Verification items for the finished model (mm, model axes). A direction names the side the tool comes from. Coordinates: 2 decimals unless noted, no trailing zeros. Write each loop counter-clockwise with the first axis right and the second up, starting at its lowest first coordinate (ties: lowest second). Pieces come first, ordered by that corner, then holes. Notation, with made-up numbers: M 4.5,54.25 L 14.5,54.25 A28 cw 14.5,73.25 Z; hole C 85.25,88 d1. An arc over 180 degrees is marked long. One line per item, written item: value.
```python
from build123d import *
from build123d.topology import SkipClean

# Parameters (mm, degrees)
BASPROSKE_W         = 26
BASPROSKE_H         = 4.375
TOOTHCUT_DEPTH      = 60.063525123
TEETHCUTS_COUNT     = 55
TEETHCUTS_ANGLE     = 353.454545455
SKETCH2_R           = 37.5
BOSS_EXTRUDE2_DEPTH = 4.5
SKETCH3_R           = 2.25
SKETCH3_R_2         = 1.8
CUT_EXTRUDE1_DEPTH  = 4.5
SKETCH4_R           = 3.25
CUT_EXTRUDE2_DEPTH  = 3
BOSS_EXTRUDE3_START = 4
SKETCH5_R           = 37.5
SKETCH5_R_2         = 28.5
BOSS_EXTRUDE3_DEPTH = 4
BOSS_EXTRUDE4_START = 7
SKETCH6_R           = 37.5
SKETCH6_R_2         = 32.75
BOSS_EXTRUDE4_DEPTH = 7
SKETCH7_R           = 1.65
BOSS_EXTRUDE5_DEPTH = 10
FILLET1_R           = 3
BOSS_EXTRUDE6_START = -10
SKETCH8_R           = 1.65
BOSS_EXTRUDE6_DEPTH = 10
FILLET2_R           = 3
SKETCH9_R           = 37.6
SKETCH9_R_2         = 37.5
BOSS_EXTRUDE7_DEPTH = 10
FILLET3_R           = 3
SKETCH10_R          = 45.899134002
SKETCH10_R_2        = 2.25
CUT_EXTRUDE3_DEPTH  = 31.5
SKETCH12_R          = 1.65
SKETCH12_R_2        = 28.5
BOSS_EXTRUDE8_DEPTH = 1.15


with BuildPart() as part:
    # BasProSke → Base-Revolve (revolve)
    with BuildSketch(Plane(origin=(0, 0, 0), x_dir=(1, 0, 0), z_dir=(0, 1, 0)), mode=Mode.PRIVATE) as base_revolve_sk:
        with Locations((13, 35.3125)):
            Rectangle(BASPROSKE_W, BASPROSKE_H)
    revolve(base_revolve_sk.sketch.rotate(Axis((-10, 0, 0), (1, 0, 0)), 180), axis=Axis((-10, 0, 0), (1, 0, 0)))

    # TooCutSke → ToothCut (cut, through all)
    with BuildSketch(Plane(origin=(0, 0, 0), x_dir=(0, 0, -1), z_dir=(1, 0, 0))):
        with BuildLine():
            ThreePointArc((1.451447951, 33.067761022), (1.040603726, 34.522224287), (0.503573985, 35.934971761))
            ThreePointArc((0.503573985, 35.934971761), (0, 35.9385), (-0.503573985, 35.934971761))
            ThreePointArc((-0.503573985, 35.934971761), (-1.040603726, 34.522224287), (-1.451447951, 33.067761022))
            ThreePointArc((-1.451447951, 33.067761022), (0, 33.0996), (1.451447951, 33.067761022))
        make_face()
    toothcut = extrude(amount=TOOTHCUT_DEPTH, mode=Mode.SUBTRACT)

    # TeethCuts: ToothCut ×55 about axis
    teethcuts_axis = Axis((-10, 0, 0), (1, 0, 0))
    for i in range(1, TEETHCUTS_COUNT):
        add(toothcut.rotate(teethcuts_axis, i * TEETHCUTS_ANGLE / (TEETHCUTS_COUNT - 1)), mode=Mode.SUBTRACT)

    # Sketch2 → Boss-Extrude2 (add)
    with BuildSketch(Plane.ZY):
        Circle(SKETCH2_R)
    extrude(amount=BOSS_EXTRUDE2_DEPTH)

    # Sketch3 → Cut-Extrude1 (cut)
    with BuildSketch(Plane.ZY.offset(4.5)):
        Circle(SKETCH3_R)
        with Locations((0, 8.5)):
            Circle(SKETCH3_R_2)
        with Locations(Location((0, -8.5, 0), (0, 0, 180))):
            Circle(SKETCH3_R_2)
    extrude(amount=-CUT_EXTRUDE1_DEPTH, mode=Mode.SUBTRACT)

    # Sketch4 → Cut-Extrude2 (cut)
    with BuildSketch(Plane(origin=(0, 0, 0), x_dir=(0, 0, -1), z_dir=(1, 0, 0))):
        with Locations((0, -8.5)):
            Circle(SKETCH4_R)
        with Locations((0, 8.5)):
            Circle(SKETCH4_R)
    extrude(amount=-CUT_EXTRUDE2_DEPTH, mode=Mode.SUBTRACT)

    # Sketch5 → Boss-Extrude3 (add)
    with BuildSketch(Plane(origin=(26, 0, 0), x_dir=(0, 0, -1), z_dir=(1, 0, 0)).offset(BOSS_EXTRUDE3_START)):
        with Locations(Location((0, 0, 0), (0, 0, 180))):
            Circle(SKETCH5_R)
        Circle(SKETCH5_R_2, mode=Mode.SUBTRACT)
    extrude(amount=-BOSS_EXTRUDE3_DEPTH)

    # Sketch6 → Boss-Extrude4 (add)
    with BuildSketch(Plane(origin=(30, 0, 0), x_dir=(0, 0, -1), z_dir=(1, 0, 0)).offset(BOSS_EXTRUDE4_START)):
        with Locations(Location((0, 0, 0), (0, 0, 180))):
            Circle(SKETCH6_R)
        Circle(SKETCH6_R_2, mode=Mode.SUBTRACT)
    extrude(amount=-BOSS_EXTRUDE4_DEPTH)

    # Sketch7 → Boss-Extrude5 (add)
    # profile 1 of 3: a face of its own
    with BuildSketch(Plane(origin=(37, 0, 0), x_dir=(0, 0, -1), z_dir=(1, 0, 0))):
        with BuildLine():
            ThreePointArc((-30.713496008, 21.515835168), (-39.750566034, 22.95), (-33.990007843, 15.840750198))
            ThreePointArc((-33.990007843, 15.840750198), (-32.475952642, 18.75), (-30.713496008, 21.515835168))
        make_face()
        with Locations((-35.507041555, 20.5)):
            Circle(SKETCH7_R, mode=Mode.SUBTRACT)
    # profile 2 of 3: a face of its own
    with BuildSketch(Plane(origin=(37, 0, 0), x_dir=(0, 0, -1), z_dir=(1, 0, 0))):
        with BuildLine():
            ThreePointArc((-3.276511835, -37.356585366), (0, -45.9), (3.276511835, -37.356585366))
            ThreePointArc((3.276511835, -37.356585366), (0, -37.5), (-3.276511835, -37.356585366))
        make_face()
        with Locations((0, -41)):
            Circle(SKETCH7_R, mode=Mode.SUBTRACT)
    # profile 3 of 3: a face of its own
    with BuildSketch(Plane(origin=(37, 0, 0), x_dir=(0, 0, -1), z_dir=(1, 0, 0))):
        with BuildLine():
            ThreePointArc((30.713496008, 21.515835168), (32.475952642, 18.75), (33.990007843, 15.840750198))
            ThreePointArc((33.990007843, 15.840750198), (39.750566034, 22.95), (30.713496008, 21.515835168))
        make_face()
        with Locations((35.507041555, 20.5)):
            Circle(SKETCH7_R, mode=Mode.SUBTRACT)
    extrude(amount=-BOSS_EXTRUDE5_DEPTH)

    # Fillet1
    fillet1_edges = [part.edges().sort_by_distance(p)[0] for p in [
        (32, 15.840750198, 33.990007843),
        (32, 21.515835168, 30.713496008),
        (32, -37.356585366, -3.276511835),
        (32, -37.356585366, 3.276511835),
        (32, 21.515835168, -30.713496008),
        (32, 15.840750198, -33.990007843),
    ]]
    fillet(fillet1_edges, radius=FILLET1_R)

    # Sketch8 → Boss-Extrude6 (add)
    # profile 1 of 3: a face of its own
    with BuildSketch(Plane.ZY.offset(4.5).offset(BOSS_EXTRUDE6_START)):
        with BuildLine():
            ThreePointArc((3.277032239, 37.357537298), (-0.001858552, 45.899133961), (-3.279499265, 37.357057531))
            ThreePointArc((-3.279499265, 37.357057531), (-0.001244018, 37.500865925), (3.277032239, 37.357537298))
        make_face()
        with Locations((0, 41)):
            Circle(SKETCH8_R, mode=Mode.SUBTRACT)
    # profile 2 of 3: a face of its own
    with BuildSketch(Plane.ZY.offset(4.5).offset(BOSS_EXTRUDE6_START)):
        with BuildLine():
            ThreePointArc((30.71426819, -21.517740103), (39.750655671, -22.948112687), (33.993202634, -15.837979147))
            ThreePointArc((33.993202634, -15.837979147), (32.478138639, -18.749677793), (30.71426819, -21.517740103))
        make_face()
        with Locations((35.507041555, -20.5)):
            Circle(SKETCH8_R, mode=Mode.SUBTRACT)
    # profile 3 of 3: a face of its own
    with BuildSketch(Plane.ZY.offset(4.5).offset(BOSS_EXTRUDE6_START)):
        with BuildLine():
            ThreePointArc((-30.712203543, -21.517680022), (-32.47526663, -18.751188157), (-33.989800256, -15.841195617))
            ThreePointArc((-33.989800256, -15.841195617), (-39.748976395, -22.951021278), (-30.712203543, -21.517680022))
        make_face()
        with Locations((-35.507041555, -20.5)):
            Circle(SKETCH8_R, mode=Mode.SUBTRACT)
    extrude(amount=BOSS_EXTRUDE6_DEPTH)


with BuildPart() as boss_extrude6_piece_1:
    # of the separate pieces the step leaves, piece 1, a body of its own (boss_extrude6_pieces)
    add(part.part.solids().sort_by_distance((37, -36.798102981, 7.221469172))[0])

    # Fillet2
    fillet2_edges = [boss_extrude6_piece_1.edges().sort_by_distance(p)[0] for p in [
        (0.5, -21.517680022, -30.712203543),
        (0.5, -15.841195617, -33.989800256),
    ]]
    fillet(fillet2_edges, radius=FILLET2_R)



with BuildPart() as boss_extrude6_piece_2:
    # of the separate pieces the step leaves, piece 2, a body of its own (boss_extrude6_pieces)
    add(part.part.solids().sort_by_distance((5.5, 37.357057531, -3.279499265))[0])


with BuildPart() as boss_extrude6_piece_3:
    # of the separate pieces the step leaves, piece 3, a body of its own (boss_extrude6_pieces)
    add(part.part.solids().sort_by_distance((5.5, -15.837979147, 33.993202634))[0])


with BuildPart() as boss_extrude6_piece_1_1:
    add(boss_extrude6_piece_1.part)

    add(boss_extrude6_piece_2.part)  # Boss-Extrude7 merges Boss-Extrude6 piece 2

    add(boss_extrude6_piece_3.part)  # Boss-Extrude7 merges Boss-Extrude6 piece 3
    # Sketch9 → Boss-Extrude7 (add)
    with BuildSketch(Plane.ZY.offset(4.5)):
        Circle(SKETCH9_R)
        Circle(SKETCH9_R_2, mode=Mode.SUBTRACT)
    extrude(amount=-BOSS_EXTRUDE7_DEPTH)

    # Fillet3
    fillet3_edges = [boss_extrude6_piece_1_1.edges().sort_by_distance(p)[0] for p in [
        (0.5, 37.448219223, 3.375037342),
        (0.5, 37.447972163, -3.377777505),
        (0.5, -21.646977688, 30.743590502),
        (0.5, -15.798744954, 34.119783966),
    ]]
    fillet(fillet3_edges, radius=FILLET3_R)

    # Sketch10 → Cut-Extrude3 (cut)
    with BuildSketch(Plane.ZY.offset(4.5)):
        Circle(SKETCH10_R)
        Circle(SKETCH10_R_2, mode=Mode.SUBTRACT)
    extrude(amount=-CUT_EXTRUDE3_DEPTH, mode=Mode.SUBTRACT)

    # Sketch12 → Boss-Extrude8 (add)
    with SkipClean():  # the faces are left unmerged after this step: merging them gives an invalid solid
        with BuildSketch(Plane.ZY.offset(-27)):
            with BuildLine():
                ThreePointArc((-32.412539248, 24.299217745), (-39.750566034, 22.95), (-37.250009483, 15.920473518))
                ThreePointArc((-37.250009483, 15.920473518), (-35.60116111, 14.39084752), (-35.478826578, 12.145075735))
                ThreePointArc((-35.478826578, 12.145075735), (-32.475952642, -18.75), (-7.221469172, -36.798102981))
                ThreePointArc((-7.221469172, -36.798102981), (-5.33774102, -38.026933686), (-4.837470235, -40.219691263))
                ThreePointArc((-4.837470235, -40.219691263), (0, -45.9), (4.837470235, -40.219691263))
                ThreePointArc((4.837470235, -40.219691263), (5.33774102, -38.026933686), (7.221469172, -36.798102981))
                ThreePointArc((7.221469172, -36.798102981), (32.475952642, -18.75), (35.478826578, 12.145075735))
                ThreePointArc((35.478826578, 12.145075735), (35.60116111, 14.39084752), (37.250009483, 15.920473518))
                ThreePointArc((37.250009483, 15.920473518), (39.750566034, 22.95), (32.412539248, 24.299217745))
                ThreePointArc((32.412539248, 24.299217745), (30.26342009, 23.636086166), (28.257357407, 24.653027246))
                ThreePointArc((28.257357407, 24.653027246), (0, 37.5), (-28.257357407, 24.653027246))
                ThreePointArc((-28.257357407, 24.653027246), (-30.177504217, 23.644648787), (-32.275580689, 24.194072128))
                add(Edge.make_bspline(
                    [(-32.275580681, 24.194072138), (-32.299145006, 24.211107976), (-32.322416857, 24.228349689), (-32.345393979, 24.245789385), (-32.368074444, 24.26341918), (-32.390456638, 24.28123123), (-32.412539248, 24.299217745)],
                    knots=[0.959340684, 0.959340684, 0.959340684, 0.959340684, 0.959340684, 0.959340684, 0.959340684, 1, 1, 1, 1, 1, 1, 1], degree=6))
            make_face()
            with Locations((0, -41)):
                Circle(SKETCH12_R, mode=Mode.SUBTRACT)
            with Locations((-35.507041555, 20.5)):
                Circle(SKETCH12_R, mode=Mode.SUBTRACT)
            Circle(SKETCH12_R_2, mode=Mode.SUBTRACT)
            with Locations((35.507041555, 20.5)):
                Circle(SKETCH12_R, mode=Mode.SUBTRACT)
        extrude(amount=BOSS_EXTRUDE8_DEPTH)


solid = boss_extrude6_piece_1_1.part
```
Item 1: Cross-section at D-D, the plane z = 13. Enter the section's corners in (x, y).
The answers:
outline: M 25.85,-35.17 L 37,-35.17 L 37,-30.06 L 30,-30.06 L 30,-25.36 L 25.85,-25.36 Z; M 25.85,25.36 L 30,25.36 L 30,30.06 L 37,30.06 L 37,35.17 L 25.85,35.17 Z
Item 2: Cross-section at B-B, the plane y = 0. Enter the section's corners in (x, z), and give its area (3 significant figures).
The answers:
outline: M 25.85,-37.5 L 37,-37.5 L 37,-32.75 L 30,-32.75 L 30,-28.5 L 25.85,-28.5 Z; M 25.85,28.5 L 30,28.5 L 30,32.75 L 37,32.75 L 37,37.5 L 25.85,37.5 Z
area: 141 mm²
Item 3: Access from +Z, -Z, +X, -X, +Y, -Y to the whole of each face (thin tool, end or side, straight path). Record for faces 3 (the face through (26.433, -38.001, -5.356)), 4 (the face through (33.549, 9.837, -31.238)), 5 (the face through (25.85, -29, 3)).
The answers:
face 3: -Z, +X, -X
face 4: +X
face 5: +Z, -Z, -X, +Y, -Y
Item 4: Go/stop test with flat-tipped pins: P1, Ø2.5, axis at y = 20.5, z = 35.51, coming from the -X side; P2, Ø1, axis at y = -25.5, z = -17.5, coming from the +X side; P3, Ø6, axis at x = 27, z = 7.5, coming from the +Y side. Record where each tip stops, or that it passes through.
The answers:
P1: passes through
P2: stops at x = 30
P3: stops at y = 37.23
Item 5: Cross-section at C-C, the plane y = 20.5. Enter the section's corners in (x, z).
The answers:
outline: M 25.85,-40.41 L 37,-40.41 L 37,-37.16 L 25.85,-37.16 Z; M 25.85,-33.86 L 37,-33.86 L 37,-25.54 L 30,-25.54 L 30,-19.8 L 25.85,-19.8 Z; M 25.85,19.8 L 30,19.8 L 30,25.54 L 37,25.54 L 37,33.86 L 25.85,33.86 Z; M 25.85,37.16 L 37,37.16 L 37,40.41 L 25.85,40.41 Z
Item 6: Draft check along Y on faces 1 (the face through (37, 33, 3)), 2 (the face through (30, 29, -3)). Enter one of: released by +Y, released by -Y, zero draft, split by the parting line, or undercut.
The answers:
face 1: zero draft
face 2: undercut
Item 7: Scan lines: line 1 (Y direction, x = 31.5, z = 0); line 2 (Z direction, x = 27.75, y = 0); line 3 (Z direction, x = 30.5, y = 20.5). Record each from-to range of solid material in increasing order.
The answers:
line 1: y = -45.9 to -42.65, -39.35 to -32.75, 32.75 to 37.5
line 2: z = -37.5 to -28.5, 28.5 to 37.5
line 3: z = -40.41 to -37.16, -33.86 to -25.54, 25.54 to 33.86, 37.16 to 40.41
